Design review of the part shown in the three views and the two pictorial views. Dimensions are in mm from the part's minimum x, y and z. A direction names the side the tool comes from. Round coordinates to 2 decimals unless told otherwise and drop trailing zeros. Loops run counter-clockwise (first coordinate to the right, second up) from the corner with the lowest first, then second, coordinate; pieces in that order, holes last. Notation, with made-up numbers: M 62.5,65.25 L 95.5,65.25 A20 cw 95.5,99.25 Z; hole C 84.5,-25.75 d4. An arc over 180 degrees is marked long. One line per question, with ' | ' between items. Start each with the question number.
1) For probe 1 along X at (y, z) = (11, 42.5) (1 decimal); probe 2 along X at (y, z) = (13.5, 32.5), list the stretches that pass through material, from the lowest coordinate up. Write a range as from..to.
2) We need section B-B (x = 41.5). Give the boundary of the cut face in (y, z) (1 decimal).
3) For pin 1 Ø3 at (y, z) = (8, 38.5) entering from +X; pin 2 Ø1.8 at (x, y) = (28.5, 9) entering from +Z; pin 3 Ø8 at (x, z) = (66.5, 48) entering from +Y, all flat-tipped, find the tip position at first contact; note any pin that passes through.
4) We need section A-A (y = 9.75). Give the boundary of the cut face in (x, z) (1 decimal).
5) We need section C-C (z = 28.5). Give the boundary of the cut face in (x, y) (1 decimal).
6) For the marked faces 1, 2 and 3, list the 3-axis set-ups (+Z, -Z, +X, -X, +Y, -Y) from which the entire face can be reached by the end or side of a thin tool; tool diameter is ignored.
7) We need section D-D (y = 1.25). Give the boundary of the cut face in (x, z) (1 decimal), and give its area (3 significant figures).
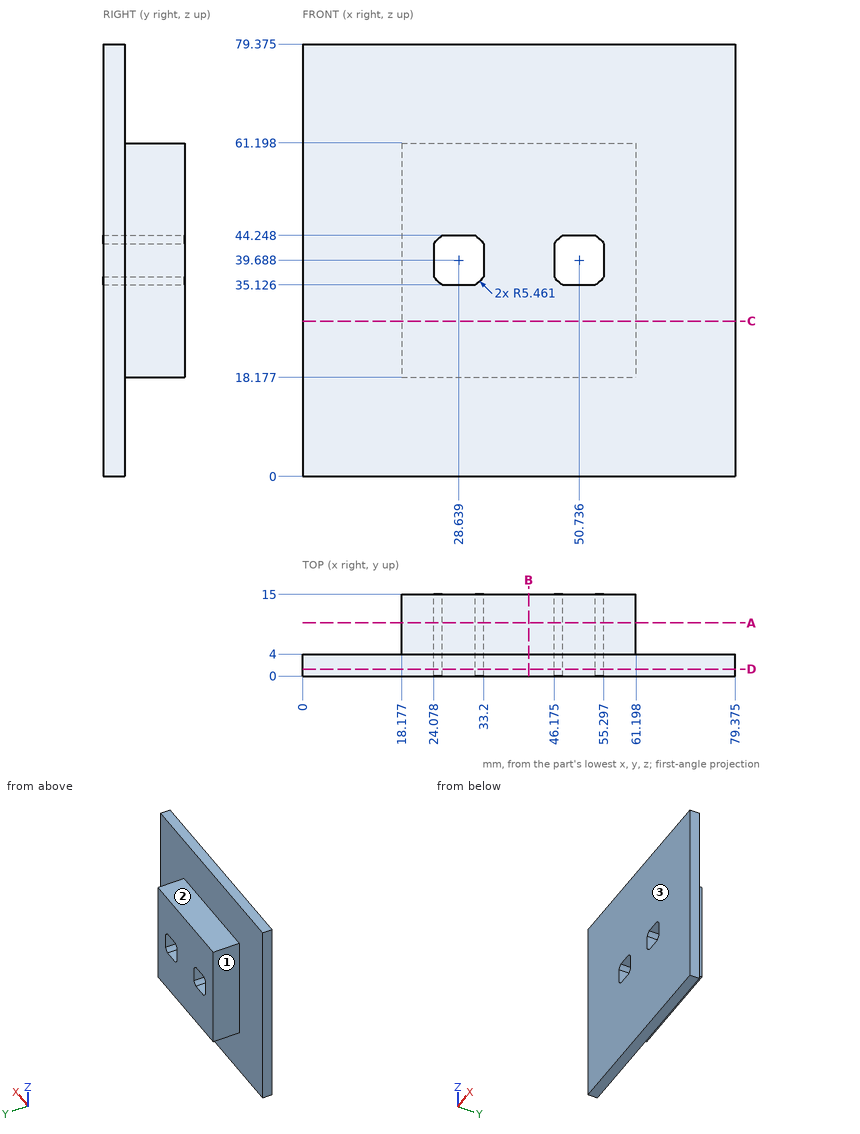
Answers below:
1) probe 1: 18.2..24.1, 33.2..46.2, 55.3..61.2 | probe 2: 18.18..61.2
2) outline: M 0,0 L 4,0 L 4,18.2 L 15,18.2 L 15,61.2 L 4,61.2 L 4,79.4 L 0,79.4 Z
3) pin 1: x = 61.2 | pin 2: z = 61.2 | pin 3: y = 4
4) outline: M 18.2,18.2 L 61.2,18.2 L 61.2,61.2 L 18.2,61.2 Z; hole M 24.1,36.7 A5.5 ccw 25.6,35.1 L 31.6,35.1 A5.5 ccw 33.2,36.7 L 33.2,42.7 A5.5 ccw 31.6,44.2 L 25.6,44.2 A5.5 ccw 24.1,42.7 Z; hole M 46.2,36.7 A5.5 ccw 47.7,35.1 L 53.7,35.1 A5.5 ccw 55.3,36.7 L 55.3,42.7 A5.5 ccw 53.7,44.2 L 47.7,44.2 A5.5 ccw 46.2,42.7 Z
5) outline: M 0,0 L 79.4,0 L 79.4,4 L 61.2,4 L 61.2,15 L 18.2,15 L 18.2,4 L 0,4 Z
6) face 1: +Z, -Z, -X, +Y | face 2: +Z, +X, -X, +Y | face 3: +Z, -Z, +X, -X, -Y
7) outline: M 0,0 L 79.4,0 L 79.4,79.4 L 0,79.4 Z; hole M 24.1,36.7 A5.5 ccw 25.6,35.1 L 31.6,35.1 A5.5 ccw 33.2,36.7 L 33.2,42.7 A5.5 ccw 31.6,44.2 L 25.6,44.2 A5.5 ccw 24.1,42.7 Z; hole M 46.2,36.7 A5.5 ccw 47.7,35.1 L 53.7,35.1 A5.5 ccw 55.3,36.7 L 55.3,42.7 A5.5 ccw 53.7,44.2 L 47.7,44.2 A5.5 ccw 46.2,42.7 Z | area: 6,140 mm^2
